Can you work these out from the model? Positions are in its coordinate system, mm. Face numbers are marked on the shaded views. Coordinates: 2 decimals unless noted, no trailing zeros. Order: outer loops, then holes, each group sorted by start corner. A loop starts at its lowest first (then second) coordinate and runs counter-clockwise, first axis right, second up. Notation, with made-up numbers: (53.5, 11.5) -> (70.5, 11.5) arc R26 cw to (70.5, 37.5) -> close; hole circle Ø1 at (-3, 6.5). An arc over 180 degrees is marked (long way). Use a Markdown table: item, result. Add a question column.
1. For pin 1 Ø6 at (x, z) = (142, -7.5) entering from +Y; pin 2 Ø12 at (x, z) = (143.5, -4) entering from -Y; pin 3 Ø4 at (x, z) = (179, 7.5) entering from -Y (3 decimals); pin 4 Ø1 at (y, z) = (6.5, -5.5) entering from +X, each with a flat end and sliding along its axis, tell me the tip position at first contact or that it passes through.
2. Suppose I cut it at D-D, the plane x = 189. List the corners of the cut face in (y, z) for me.
3. Suppose I cut it at A-A, the plane z = 0. List the corners of the cut face in (x, y) for me.
4. We'd pull the mould along Y, two halves only. Please class the marked faces 1, 2 and 3: pulls with the +Y half, pulls with the -Y half, needs draft (parallel to the pull), parting line crosses it, or undercut.
5. If I drill on line 1 along Y through (x, z) = (178.25, 0); line 2 along Y through (x, z) = (94, 0), over which ranges is the centre line in solid material (lowest first)? Write a range as from..to.
6. Suppose I cut it at C-C, the plane x = 118. List the corners of the cut face in (y, z) for me, then the cut area to 3 significant figures.
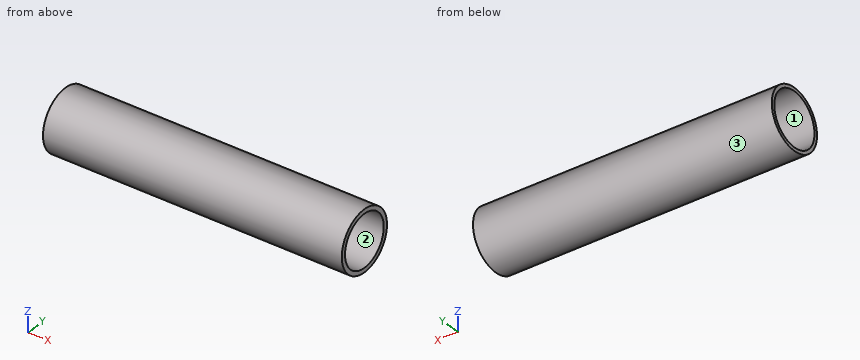
```python
from build123d import *

# Parameters (mm, degrees)
CYLINDER004_R           = 10.7
CYLINDER004_DEPTH       = 27
CYLINDER004_PITCH_ANGLE = 90
CYLINDER003_R           = 11.1
CYLINDER003_DEPTH       = 97
CYLINDER003_PITCH_ANGLE = 90
CYLINDER002_R           = 12.5
CYLINDER002_DEPTH       = 124
CYLINDER002_PITCH_ANGLE = 90


with BuildPart() as cylinder002:
    # Cylinder004 → Cylinder004 (new body)
    with BuildSketch(Plane.XY):
        Circle(CYLINDER004_R)
    extrude(amount=CYLINDER004_DEPTH)


with BuildPart() as cylinder002_1:
    # Cylinder004 pitch: moved
    add(cylinder002.part.rotate(Axis((0, 0, 0), (0, 1, 0)), CYLINDER004_PITCH_ANGLE))


with BuildPart() as cylinder002_2:
    # Cylinder004 placement: moved
    add(cylinder002_1.part.moved(Location((171, 0, 0))))


with BuildPart() as cylinder001:
    # Cylinder003 → Cylinder003 (new body)
    with BuildSketch(Plane.XY):
        Circle(CYLINDER003_R)
    extrude(amount=CYLINDER003_DEPTH)


with BuildPart() as cylinder001_1:
    # Cylinder003 pitch: moved
    add(cylinder001.part.rotate(Axis((0, 0, 0), (0, 1, 0)), CYLINDER003_PITCH_ANGLE))


with BuildPart() as cylinder001_2:
    # Cylinder003 placement: moved
    add(cylinder001_1.part.moved(Location((74, 0, 0))))


with BuildPart() as batteryholder:
    # Cylinder002 → Cylinder002 (new body)
    with BuildSketch(Plane.XY):
        Circle(CYLINDER002_R)
    extrude(amount=CYLINDER002_DEPTH)


with BuildPart() as batteryholder_1:
    # Cylinder002 pitch: moved
    add(batteryholder.part.rotate(Axis((0, 0, 0), (0, 1, 0)), CYLINDER002_PITCH_ANGLE))


with BuildPart() as batteryholder_2:
    # Cylinder002 placement: moved
    add(batteryholder_1.part.moved(Location((74, 0, 0))))

    # Cut001: cut Cylinder001
    add(cylinder001_2.part, mode=Mode.SUBTRACT)

    # Cut002: cut Cylinder002
    add(cylinder002_2.part, mode=Mode.SUBTRACT)


solid = batteryholder_2.part
```
Worked out:
| question | item | result |
|---|---|---|
| 1 | pin 1 | stops at y = 11.66 |
| 1 | pin 2 | stops at y = -12.5 |
| 1 | pin 3 | stops at y = -11.225 |
| 1 | pin 4 | passes through |
| 2 | outline | circle Ø25 at (0, 0); hole circle Ø21.4 at (0, 0) |
| 3 | outline | (74, -12.5) -> (198, -12.5) -> (198, -10.7) -> (171, -10.7) -> (171, -11.1) -> (74, -11.1) -> close; (74, 11.1) -> (171, 11.1) -> (171, 10.7) -> (198, 10.7) -> (198, 12.5) -> (74, 12.5) -> close |
| 4 | face 1 | undercut |
| 4 | face 2 | undercut |
| 4 | face 3 | parting line crosses it |
| 5 | line 1 | y = -12.5..-10.7, 10.7..12.5 |
| 5 | line 2 | y = -12.5..-11.1, 11.1..12.5 |
| 6 | outline | circle Ø25 at (0, 0); hole circle Ø22.2 at (0, 0) |
| 6 | area | 104 mm² |
